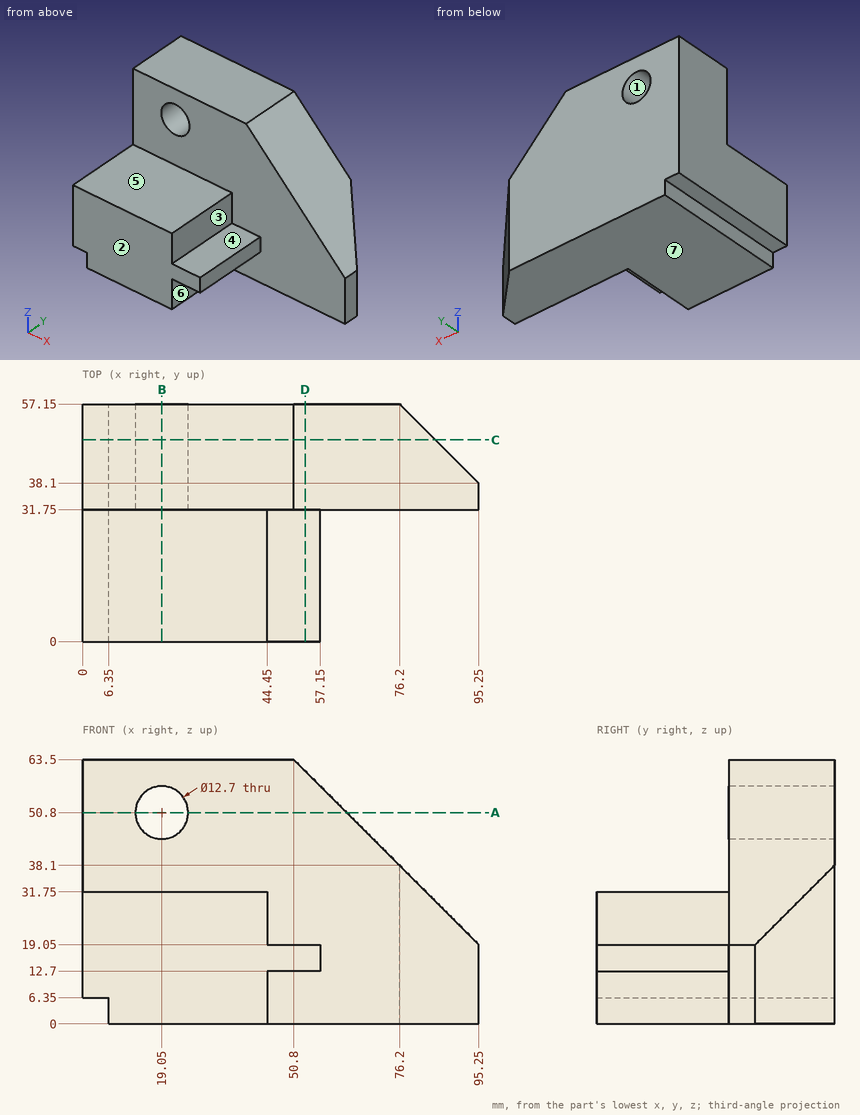
Answer from the drawing. Dimensions are ordinates in mm from the lowest x, y and z of the part. A direction names the side the tool comes from. Give positions to 0.01 mm unless a question says otherwise; leave off trailing zeros. Write each loop counter-clockwise with the first axis right and the second up, starting at its lowest first coordinate (ties: lowest second). Pieces come first, ordered by that corner, then holes. Notation, with made-up numbers: (-31.75, 20) -> (-26.75, 20) arc R18 cw to (-26.75, 28) -> close; hole circle Ø1 at (-10, 51.5). An arc over 180 degrees is marked (long way). One line per question, with ' | ' between items. Start each with the question number.
1. Section B-B (x = 19.05) is taken. Determine the outline of the cut face in (y, z).
2. For the marked faces 4, 5, 6 and 7, determine the directions among +Z, -Z, +X, -X, +Y, -Y from which every point of the face is accessible in a straight line to the end or side of a thin tool.
3. For a pull along X with two mould halves and no side action, classify the marked faces 1, 2 and 3 as pulls with the +X half, pulls with the -X half, needs draft (parallel to the pull), parting line crosses it, or undercut.
4. Find the intervals of material crossed by probe 1 along Z at (x, y) = (19.05, 43.25); probe 2 along Y at (x, z) = (65, 46); probe 3 along Z at (x, y) = (31.5, 26), in increasing order.
5. Section D-D (x = 53.5) is taken. Determine the outline of the cut face in (y, z).
6. Given pin 1 Ø1.5 at (y, z) = (45, 48.5) entering from +X; pin 2 Ø5 at (y, z) = (23, 16) entering from +X; pin 3 Ø1.5 at (x, z) = (48.5, 21.5) entering from -Y; pin 4 Ø1 at (y, z) = (34, 56.5) entering from -X, each flat-ended and moving along its own axis, determine where each tip first touches the part or whether it passes through.
7. Section C-C (y = 48.5) is taken. Determine the outline of the cut face in (x, z).
8. Section A-A (z = 50.8) is taken. Determine the outline of the cut face in (x, y), plus the area to 3 significant figures.
Response values:
1) outline: (0, 0) -> (57.15, 0) -> (57.15, 44.45) -> (31.75, 44.45) -> (31.75, 31.75) -> (0, 31.75) -> close; (31.75, 57.15) -> (57.15, 57.15) -> (57.15, 63.5) -> (31.75, 63.5) -> close
2) face 4: +Z, +X, -Y | face 5: +Z, +X, -X, -Y | face 6: -Z, +X, -Y | face 7: -Z, +X, -X, +Y, -Y
3) face 1: undercut | face 2: needs draft | face 3: pulls with the +X half
4) probe 1: 0 to 44.45, 57.15 to 63.5 | probe 2: 31.75 to 57.15 | probe 3: 0 to 31.75
5) outline: (0, 12.7) -> (31.75, 12.7) -> (31.75, 0) -> (57.15, 0) -> (57.15, 60.8) -> (31.75, 60.8) -> (31.75, 19.05) -> (0, 19.05) -> close
6) pin 1: x = 66.55 | pin 2: x = 57.15 | pin 3: y = 31.75 | pin 4: x = 0
7) outline: (0, 6.35) -> (6.35, 6.35) -> (6.35, 0) -> (84.85, 0) -> (84.85, 29.45) -> (50.8, 63.5) -> (0, 63.5) -> close; hole circle Ø12.7 at (19.05, 50.8)
8) outline: (0, 31.75) -> (12.7, 31.75) -> (12.7, 57.15) -> (0, 57.15) -> close; (25.4, 31.75) -> (63.5, 31.75) -> (63.5, 57.15) -> (25.4, 57.15) -> close | area: 1,290 mm2
